Geometry: final body of the model. Coordinates: model frame, mm. Face numbers are marked on the shaded views. A direction names the side the tool comes from. Give positions to 0.01 mm unless a question says otherwise; leave off trailing zeros. Write each loop counter-clockwise with the first axis right and the second up, starting at its lowest first coordinate (ties: lowest second). Pieces come first, ordered by that corner, then holes. Notation, with made-up numbers: M 55.25,3 L 76.25,3 A34 ccw 76.25,39 Z; hole C -8.75,78.5 d6. An arc over 180 degrees is marked long. Answer as a JSON object with one key per item and string values.
Autodesk Inventor part; units mm, degrees
ref_plane "YZ Plane" through (0, 0, 0) normal (1, 0, 0) x (0, 1, 0)
ref_plane "XZ Plane" through (0, 0, 0) normal (0, 1, 0) x (-1, 0, 0)
ref_plane "XY Plane" through (0, 0, 0) normal (0, 0, 1) x (1, 0, 0)
sketch "Sketch1" plane through (0, 0, 0) normal (0, 1, 0) x (-1, 0, 0)
  point P0 (0, 0)
sketch "Sketch2" plane through (0, 0, 0) normal (0, 0, 1) x (1, 0, 0)
  line L0 (0, 0) -> (50.8, 0)
  line L1 (50.8, 0) -> (50.8, 25.4)
  line L2 (50.8, 25.4) -> (0, 25.4)
  line L3 (0, 25.4) -> (0, 0)
  line L4 (6.35, 0) -> (44.45, 0)
  line L5 (44.45, 0) -> (44.45, 19.05)
  line L6 (44.45, 19.05) -> (6.35, 19.05)
  line L7 (6.35, 19.05) -> (6.35, 0)
  dimension "d0" = 6.35
  dimension "d1" = 6.35
  dimension "d2" = 6.35
  dimension "d3" = 38.1
  dimension "d4" = 25.4
extrude "Extrusion1" add sketch "Sketch2" along normal blind 50.8 contours L3 L2 L1 L0 L5 L6 L7
ref_plane "Work Plane1" through (25.4, 0, 0) normal (1, 0, 0) x (0, 0, -1)
sketch "Sketch4" plane through (0, 0, 0) normal (0, -1, 0) x (1, 0, 0)
  circle A0 centre (3.175, 44.45) radius 1.651
  line L0 (6.35, 0) -> (6.35, 50.8)
  line L1 (0, 50.8) -> (6.35, 50.8)
  circle A1 centre (3.175, 6.35) radius 1.651
  line L2 (0, 0) -> (6.35, 0)
  line L3 (50.8, 50.8) -> (0, 50.8)
  line L4 (25.4, 50.8) -> (25.4, 0)
  line L5 (50.8, 0) -> (0, 0)
  circle A2 centre (47.625, 44.45) radius 1.651
  circle A3 centre (47.625, 6.35) radius 1.651
  dimension "d13" = 3.302
  dimension "d14" = 3.175
  dimension "d15" = 6.35
  dimension "d16" = 3.302
  dimension "d17" = 6.35
extrude "Extrusion2" cut sketch "Sketch4" against normal blind 12.7 contours A0 | A1 | A2 | A3
properties part number "WIREBRIDGE" material "ABS Plastic"
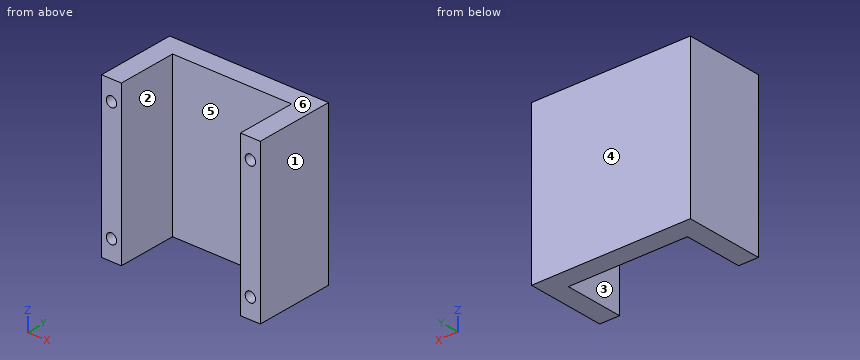
1) Cut plane A-A on y = 9.5. Return loops of the section in (x, z) (3 decimals).
Geometry check:
{"outline": "M 0,0 L 6.35,0 L 6.35,50.8 L 0,50.8 Z; M 44.45,0 L 50.8,0 L 50.8,50.8 L 44.45,50.8 Z; hole C 3.175,6.35 d3.302; hole C 3.175,44.45 d3.302; hole C 47.625,6.35 d3.302; hole C 47.625,44.45 d3.302"}
2) Line query: line 1 (Z direction, x = 3, y = 10); line 2 (X direction, y = 7.25, z = 43); line 3 (X direction, y = 6.25, z = 30). Output: solid intervals per line, ascending. Write a range as from..to.
Geometry check:
{"line 1": "z = 0..4.71, 7.99..42.81, 46.09..50.8", "line 2": "x = 0..2.39, 3.96..6.35, 44.45..46.84, 48.41..50.8", "line 3": "x = 0..6.35, 44.45..50.8"}
3) Contact query for flat-ended pins moving along their axis: P1, Ø1, axis at x = 48.5, z = 6.5, coming from the -Y side; P2, Ø19, axis at x = 31, z = 20.5, coming from the -Y side. Output: stop coordinate, or through.
Geometry check:
{"P1": "stops at y = 12.7", "P2": "stops at y = 19.05"}
4) Cut plane B-B on z = 6.35. Return loops of the section in (x, y), and give its area (3 significant figures).
Geometry check:
{"outline": "M 0,0 L 1.52,0 L 1.52,12.7 L 4.83,12.7 L 4.83,0 L 6.35,0 L 6.35,19.05 L 44.45,19.05 L 44.45,0 L 45.97,0 L 45.97,12.7 L 49.28,12.7 L 49.28,0 L 50.8,0 L 50.8,25.4 L 0,25.4 Z", "area": "481 mm2"}
5) Set-up query: the marked faces 5 and 6. Return all of +Z, -Z, +X, -X, +Y, -Y with unobstructed straight access to the full face (end or side cutting, diameter ignored); none if empty.
Geometry check:
{"face 5": "+Z, -Z, -Y", "face 6": "+Z, +X, -X, +Y, -Y"}
6) Pull-direction query (X, two-part tool) for the marked faces 1, 2, 3 and 4; classes: pulls with the +X half, pulls with the -X half, needs draft (parallel to the pull), parting line crosses it, or undercut.
Geometry check:
{"face 1": "pulls with the +X half", "face 2": "undercut", "face 3": "undercut", "face 4": "needs draft"}
7) Cut plane C-C on x = 14. Return loops of the section in (y, z), and give its area (3 significant figures).
Geometry check:
{"outline": "M 19.05,0 L 25.4,0 L 25.4,50.8 L 19.05,50.8 Z", "area": "323 mm2"}
